Read the model definition and answer for the solid it produces. Units are mm, in the model's axes. Give positions to 0.01 mm unless a question says otherwise; leave off trailing zeros. Order: outer loops, then holes, each group sorted by start corner. A loop starts at its lowest first (then second) coordinate and runs counter-clockwise, first axis right, second up.
Item 1: Given pin 1 Ø2 at (y, z) = (-3, 86) entering from -X; pin 2 Ø10 at (x, y) = (29.5, 8.5) entering from -Z; pin 3 Ø6 at (y, z) = (19.5, 28.5) entering from -X; pin 4 Ø2 at (y, z) = (-9, 55.5) entering from -X, each flat-ended and moving along its own axis, determine where each tip first touches the part or whether it passes through.
Item 2: A cutting plane is placed at A-A (y = 0). Write down the section's boundary in (x, z).
Item 3: Find the intervals of material crossed by line 1 along Y through (x, z) = (0.5, 90.5); line 2 along Z through (x, y) = (-2, -23); line 3 along Y through (x, z) = (4, 41), in increasing order.
Item 4: A cutting plane is placed at C-C (z = 64). Write down the section's boundary in (x, y), plus the area to 3 significant figures.
Item 5: A cutting plane is placed at D-D (z = 8.5). Write down the section's boundary in (x, y), plus the area to 3 significant figures.
Item 6: The mould has two halves that part along X. Classify faces 1 (the face through (-33.727, -25.861, 55.63)), 2 (the face through (-1, 1, 0)), 3 (the face through (20.765, -39.923, 47.165)), 4 (the face through (-1, 1, 10)): +X half, -X half, draft (parallel to the pull), parting line (faces both ways), or undercut.
from build123d import *

# Parameters (mm, degrees)
F0_R     = 45
F1_DEPTH = 100
F3_R     = 42.5
F4_DEPTH = 90


# Not quite as in the source:
# - a fillet or chamfer that OpenCascade refuses, or shapes differently, is made with other operations: its cross-section is extruded or revolved along the edge and cut away or added


with BuildPart() as f1:
    # F0 (on Top) → F1 (new body)
    with BuildSketch(Plane.XY):
        Circle(F0_R)
    extrude(amount=F1_DEPTH)

    # F3 (on face) → F4 (cut)
    with BuildSketch(Plane.XY.offset(100)):
        Circle(F3_R)
    extrude(amount=-F4_DEPTH, mode=Mode.SUBTRACT)

    # F5: fillet of radius 5 on 1 edges, made by hand

    # F5_s1 → F5_t2 (revolve, cut)
    with BuildSketch(Plane.XZ):
        with BuildLine():
            ThreePointArc((45, 95.6698729811), (44.3301270189, 98.1698729811), (42.5, 100))
            Line((42.5, 100), (45, 100))
            Line((45, 100), (45, 95.6698729811))
        make_face()
    revolve(axis=Axis((0, 0, 100), (0, 0, 1)), mode=Mode.SUBTRACT)


solid = f1.part
Response values:
1. pin 1: stops at x = -44.96
1. pin 2: stops at z = 0
1. pin 3: stops at x = -41.87
1. pin 4: stops at x = -44.28
2. outline: (-45, 0) - (45, 0) - (45, 95.67) arc R5 ccw to (42.5, 100) - (42.5, 10) - (-42.5, 10) - (-42.5, 100) arc R5 ccw to (-45, 95.67) - close
3. line 1: y = -45 to -42.5, 42.5 to 45
3. line 2: z = 0 to 10
3. line 3: y = -44.82 to -42.31, 42.31 to 44.82
4. outline: circle Ø90 at (0, 0); hole circle Ø85 at (0, 0)
4. area: 687 mm2
5. outline: circle Ø90 at (0, 0)
5. area: 6,360 mm2
6. face 1: undercut
6. face 2: draft
6. face 3: parting line
6. face 4: undercut
